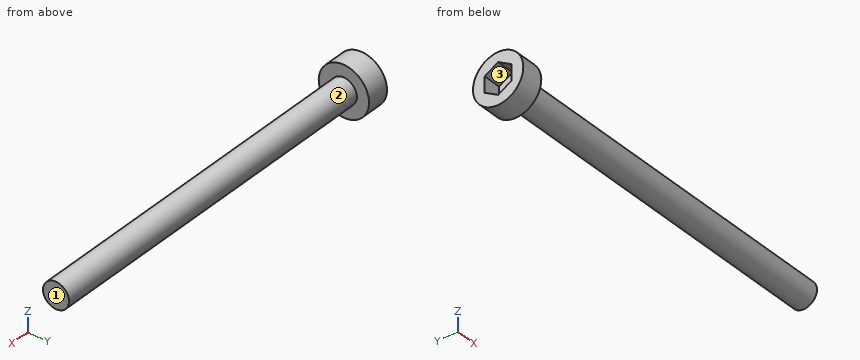
```python
from build123d import *

# Parameters (mm, degrees)
IZIM1_R                     = 1.45
Y_KSEKLIK_EKSTR_ZYON1_DEPTH = 40
IZIM2_R                     = 2.8
Y_KSEKLIK_EKSTR_ZYON2_DEPTH = 2.5
KES_EKSTR_ZYON1_DEPTH       = 2


with BuildPart() as part:
    # Çizim1 → Yükseklik-Ekstrüzyon1 (new body)
    with BuildSketch(Plane(origin=(0, 0, 0), x_dir=(0, 0, -1), z_dir=(1, 0, 0))):
        Circle(IZIM1_R)
    extrude(amount=Y_KSEKLIK_EKSTR_ZYON1_DEPTH)

    # Çizim2 → Yükseklik-Ekstrüzyon2 (add)
    with BuildSketch(Plane.ZY):
        Circle(IZIM2_R)
    extrude(amount=Y_KSEKLIK_EKSTR_ZYON2_DEPTH)

    # Çizim3 → Kes-Ekstrüzyon1 (cut)
    with BuildSketch(Plane.ZY.offset(2.5)):
        Polygon((0.866025404, -1.5), (1.732050808, 0), (0.866025404, 1.5), (-0.866025404, 1.5), (-1.732050808, 0), (-0.866025404, -1.5), align=None)
    extrude(amount=-KES_EKSTR_ZYON1_DEPTH, mode=Mode.SUBTRACT)


solid = part.part
```
Build history of the part. All positions in model axes, mm. Face numbers are marked on the shaded views. Round coordinates to 2 decimals unless told otherwise and drop trailing zeros. Write each loop counter-clockwise with the first axis right and the second up, starting at its lowest first coordinate (ties: lowest second). Pieces come first, ordered by that corner, then holes. Notation, with made-up numbers: (75.5, 73) - (125.5, 73) arc R7 ccw to (125.5, 85) - close; hole circle Ø9 at (-35, 71.25). An arc over 180 degrees is marked (long way). Write each question's results on one line, items separated by ' | '. Start each with the question number.
Item 1: Saw through at A-A (z = 0). Write the cut outline in (x, y).
Item 2: Drop flat-ended pins along their axis: P1, Ø1.5, axis at y = 0, z = -0.5, coming from the -X side; P2, Ø2, axis at x = 8.5, z = 0, coming from the +Y side; P3, Ø2, axis at x = 21, z = 0, coming from the -Y side. Give the stop position or say it passes through.
Item 3: Saw through at B-B (x = 23). Write the cut outline in (y, z).
Item 4: Saw through at C-C (z = -2.1). Write the cut outline in (x, y), and give its area (3 significant figures).
Item 5: Wall check: L1, parallel to Y at x = 5, z = -0.05; L2, parallel to X at y = -0.65, z = -1.25; L3, parallel to X at y = -1.4, z = 1.6. Give the ranges that are in metal, low to high. Write a range as [from, to].
Item 6: Mould opens along Y. For the marked faces 1, 2 and 3 say: pulls with the +Y half, pulls with the -Y half, needs draft (parallel to the pull), parting line crosses it, or undercut.
Results are:
1) outline: (-2.5, -2.8) - (0, -2.8) - (0, -1.45) - (40, -1.45) - (40, 1.45) - (0, 1.45) - (0, 2.8) - (-2.5, 2.8) - (-2.5, 1.5) - (-0.5, 1.5) - (-0.5, -1.5) - (-2.5, -1.5) - close
2) P1: stops at x = -0.5 | P2: stops at y = 1.45 | P3: stops at y = -1.45
3) outline: circle Ø2.9 at (0, 0)
4) outline: (-2.5, -1.85) - (0, -1.85) - (0, 1.85) - (-2.5, 1.85) - close | area: 9.26 mm²
5) L1: y = [-1.45, 1.45] | L2: x = [-0.5, 40] | L3: x = [-2.5, 0]
6) face 1: needs draft | face 2: parting line crosses it | face 3: undercut
